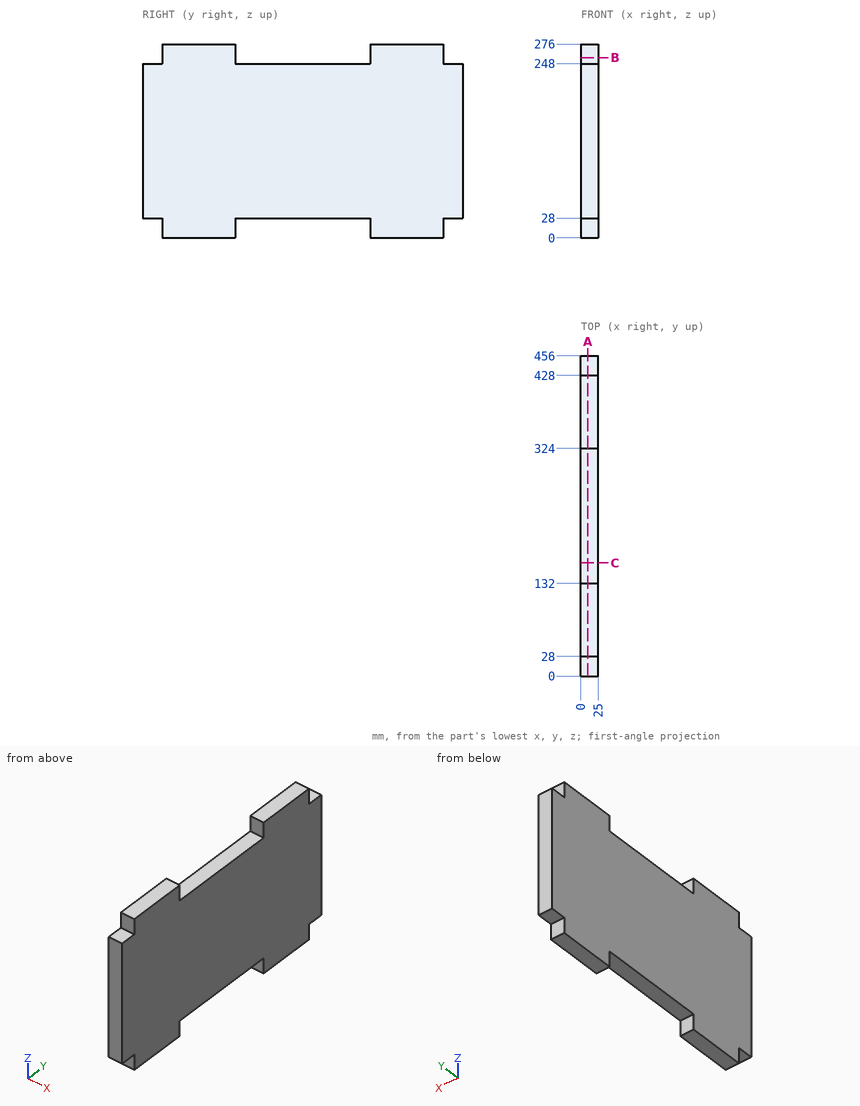
The drawing under review shows one solid part. Ordinate dimensions are in mm from its lowest x, y, z. Coordinates: 2 decimals unless noted, no trailing zeros. Write each loop counter-clockwise with the first axis right and the second up, starting at its lowest first coordinate (ties: lowest second). Pieces come first, ordered by that corner, then holes. Notation, with made-up numbers: (32, 57.5) - (40, 57.5) arc R21 cw to (40, 82.5) - close; hole circle Ø3 at (-23.75, 2.5). An arc over 180 degrees is marked (long way). Answer as CSV lines item,"result".
(1) Clearance check with flat-ended pins moving along their axes: pin 1 Ø7.5 at (x, y) = (15.5, 8.5) entering from +Z; pin 2 Ø12.5 at (x, z) = (18.5, 11.5) entering from -Y; pin 3 Ø7.5 at (x, z) = (10, 265.5) entering from +Y. State where each tip first meets the part, or that it passes through.
Data:
pin 1,"stops at z = 248"
pin 2,"stops at y = 28"
pin 3,"stops at y = 428"
(2) We need section C-C (y = 161). Give the boundary of the cut face in (x, z), plus the area to 3 significant figures.
Data:
outline,"(0, 28) - (25, 28) - (25, 248) - (0, 248) - close"
area,"5,500 mm2"
(3) We need section A-A (x = 10). Give the boundary of the cut face in (y, z), plus the area to 3 significant figures.
Data:
outline,"(0, 28) - (28, 28) - (28, 0) - (132, 0) - (132, 28) - (324, 28) - (324, 0) - (428, 0) - (428, 28) - (456, 28) - (456, 248) - (428, 248) - (428, 276) - (324, 276) - (324, 248) - (132, 248) - (132, 276) - (28, 276) - (28, 248) - (0, 248) - close"
area,"112,000 mm2"
(4) For line 1 along Y through (x, z) = (18, 26.5); line 2 along Z through (x, y) = (15, 25), list the stretches that pass through material, from the lowest coordinate up. Write a range as [from, to].
Data:
line 1,"y = [28, 132], [324, 428]"
line 2,"z = [28, 248]"
(5) We need section B-B (z = 256.5). Give the boundary of the cut face in (x, y), plus the area to 3 significant figures.
Data:
outline,"(0, 28) - (25, 28) - (25, 132) - (0, 132) - close; (0, 324) - (25, 324) - (25, 428) - (0, 428) - close"
area,"5,200 mm2"
